```python
from build123d import *

# Parameters (mm, degrees)
F1_DEPTH = 38
F2_R     = 20.15
F3_DEPTH = 26
F5_DEPTH = 93
F7_DEPTH = 34.501


with BuildPart() as f1:
    # F0 (on Top) → F1 (new body)
    with BuildSketch(Plane.XY):
        with BuildLine():
            Line((9.380832, 21), (-9.380832, 21))
            ThreePointArc((-9.380832, 21), (-23, 0), (-9.380832, -21))
            Line((-9.380832, -21), (9.380832, -21))
            ThreePointArc((9.380832, -21), (23, 0), (9.380832, 21))
        make_face()
    extrude(amount=F1_DEPTH)

    # F2 (on face) → F3 (cut)
    with BuildSketch(Plane.XY.offset(38)):
        Circle(F2_R)
    extrude(amount=-F3_DEPTH, mode=Mode.SUBTRACT)

    # F4 (on face) → F5 (join)
    with BuildSketch(Plane(origin=(0, 0, 0), x_dir=(1, 0, 0), z_dir=(0, 0, -1))):
        with BuildLine():
            Line((-11.5, 15.748016), (-11.5, -15.748016))
            ThreePointArc((-11.5, -15.748016), (0, -19.5), (11.5, -15.748016))
            Line((11.5, -15.748016), (11.5, 15.748016))
            ThreePointArc((11.5, 15.748016), (0, 19.5), (-11.5, 15.748016))
        make_face()
    extrude(amount=F5_DEPTH)

    # F6 (on face) → F7 (cut, through all)
    with BuildSketch(Plane(origin=(-11.5, 0, 0), x_dir=(0, -1, 0), z_dir=(-1, 0, 0))):
        with BuildLine():
            Line((15.748016, -93), (15.748016, -86.763055))
            ThreePointArc((15.748016, -86.763055), (8.469054, -91.383992), (0, -93))
            Line((0, -93), (15.748016, -93))
        make_face()
        with BuildLine():
            Line((-15.748016, -93), (0, -93))
            ThreePointArc((0, -93), (-8.469054, -91.383992), (-15.748016, -86.763055))
            Line((-15.748016, -86.763055), (-15.748016, -93))
        make_face()
        with BuildLine():
            Line((22.997589, -108.386131), (22.997589, -70.332999))
            ThreePointArc((22.997589, -70.332999), (21.042627, -79.284818), (15.748016, -86.763055))
            Line((15.748016, -86.763055), (15.748016, -93))
            Line((15.748016, -93), (0, -93))
            Line((0, -93), (-15.748016, -93))
            Line((-15.748016, -93), (-15.748016, -86.763055))
            ThreePointArc((-15.748016, -86.763055), (-21.30932, -78.655224), (-22.976737, -68.96581))
            Line((-22.976737, -68.96581), (-35.855297, -106.006794))
            Line((-35.855297, -106.006794), (22.997589, -108.386131))
        make_face()
    extrude(amount=-F7_DEPTH, mode=Mode.SUBTRACT)


solid = f1.part
```
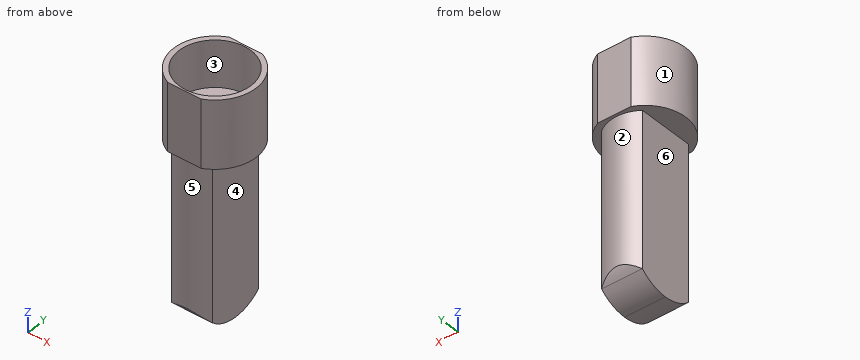
Design review of the part built by this model. Coordinates are the model's own, in mm. Face numbers are marked on the shaded views. A direction names the side the tool comes from. Coordinates: 2 decimals unless noted, no trailing zeros. Order: outer loops, then holes, each group sorted by start corner. A loop starts at its lowest first (then second) coordinate and runs counter-clockwise, first axis right, second up. Notation, with made-up numbers: (33, 58) - (68, 58) arc R22 cw to (68, 67) - close; hole circle Ø7 at (74, -37). An arc over 180 degrees is marked (long way). Answer in a Markdown table with one row per item.
(1) Clearance check with flat-ended pins moving along their axes: pin 1 (20 mm diameter, centred on x = 3, y = 5.5, fed in from +Z); pin 2 (1.5 mm diameter, centred on y = 0, z = -54, fed in from -X); pin 3 (10 mm diameter, centred on x = -1, z = -56.5, fed in from -Y). State where each tip first meets the part, or that it passes through.
Checked values:
| item | result |
|---|---|
| pin 1 | z = 12 |
| pin 2 | x = -11.5 |
| pin 3 | y = -19.5 |
(2) Consider section A-A on x = 0. State the section outline as (y, z) points.
Checked values:
| item | result |
|---|---|
| outline | (-21, 0) - (-19.5, 0) - (-19.5, -82.2) arc R23 ccw to (-15.75, -86.76) arc R23 ccw to (0, -93) arc R23 ccw to (15.75, -86.76) arc R23 ccw to (19.5, -82.2) - (19.5, 0) - (21, 0) - (21, 38) - (20.15, 38) - (20.15, 12) - (-20.15, 12) - (-20.15, 38) - (-21, 38) - close |
(3) Wall thickness on line 1 along Y through (x, z) = (0, 18.25); line 2 along Z through (x, y) = (-19, 0.5); line 3 along Z through (x, y) = (-11, 1): over which ranges is each line inside the solid? List them lowest first. Write a range as from..to.
Checked values:
| item | result |
|---|---|
| line 1 | -21..-20.15, 20.15..21 |
| line 2 | 0..12 |
| line 3 | -92.98..12 |
(4) For the marked faces 4, 5 and 6, list the 3-axis set-ups (+Z, -Z, +X, -X, +Y, -Y) from which the entire face can be reached by the end or side of a thin tool; tool diameter is ignored.
Checked values:
| item | result |
|---|---|
| face 4 | -Z, +X, +Y, -Y |
| face 5 | -Z, -Y |
| face 6 | -Z, -X, +Y, -Y |
(5) Consider section C-C on z = -33. State the section outline as (x, y) points, plus the area to 3 significant figures.
Checked values:
| item | result |
|---|---|
| outline | (-11.5, -15.75) arc R19.5 ccw to (11.5, -15.75) - (11.5, 15.75) arc R19.5 ccw to (-11.5, 15.75) - close |
| area | 842 mm^2 |
(6) Consider section D-D on y = -3. State the section outline as (x, z) points, plus the area to 3 significant figures.
Checked values:
| item | result |
|---|---|
| outline | (-22.8, 0) - (-11.5, 0) - (-11.5, -92.8) - (11.5, -92.8) - (11.5, 0) - (22.8, 0) - (22.8, 38) - (19.93, 38) - (19.93, 12) - (-19.93, 12) - (-19.93, 38) - (-22.8, 38) - close |
| area | 2,830 mm^2 |
(7) Consider section B-B on y = -8.5. State the section outline as (x, z) points.
Checked values:
| item | result |
|---|---|
| outline | (-21.37, 0) - (-11.5, 0) - (-11.5, -91.37) - (11.5, -91.37) - (11.5, 0) - (21.37, 0) - (21.37, 38) - (18.27, 38) - (18.27, 12) - (-18.27, 12) - (-18.27, 38) - (-21.37, 38) - close |
(8) The part is to be moulded in two halves that separate along X. For the marked faces 1, 2 and 3, say which applies: released by +X, released by -X, zero draft, split by the parting line, or undercut.
Checked values:
| item | result |
|---|---|
| face 1 | released by -X |
| face 2 | split by the parting line |
| face 3 | undercut |
